Check sheet for the modelled part. Datum: model origin and axes. Units: mm. A direction names the side the tool comes from. Coordinates: 2 decimals unless noted, no trailing zeros. Order: outer loops, then holes, each group sorted by start corner. A loop starts at its lowest first (then second) coordinate and runs counter-clockwise, first axis right, second up.
from build123d import *

# Parameters (mm, degrees)
SKETCH1_W             = 140
SKETCH1_H             = 14
SKETCH1_W_2           = 180
SKETCH1_H_2           = 90
BOSS_EXTRUDE1_DEPTH   = 3
BOSS_EXTRUDE2_DEPTH   = 40
BOSS_EXTRUDE2_DRAFT   = -25
SHELL1_T              = -2
BOSS_EXTRUDE4_DEPTH   = 1.5
SCALE1_SCALE          = 0.4777778
CUT_EXTRUDE3_START    = -10
CUT_EXTRUDE3_DEPTH    = 4
SNAP_START            = -31.975695848
SNAP_HOOK1_DEPTH      = 0.247222222
SNAP_START_2          = -6.313244992
SNAP_HOOK1_2_DEPTH    = 7.314130886
SNAP_START_3          = -5.262379505
SNAP_HOOK1_3_DEPTH    = 5.212399912
SNAP_START_4          = -34
SNAP_HOOK1_4_DEPTH    = 4
SKETCH16_W            = 5
SKETCH16_H            = 1
SKETCH16_W_2          = 0.5
SKETCH16_H_2          = 3.5
SKETCH16_W_3          = 10.020724484
SKETCH16_W_4          = 6.639207239
BOSS_EXTRUDE5_DEPTH   = 10
CUT_EXTRUDE8_DEPTH    = 3.5
BOSS_EXTRUDE9_DEPTH   = 1.5
MIRROR34_START        = -31.975695848
MIRROR34_COPY_1_DEPTH = 0.247222222
MIRROR34_START_2      = -6.313244992
MIRROR34_COPY_2_DEPTH = 7.314130886
MIRROR34_START_3      = -5.262379505
MIRROR34_COPY_3_DEPTH = 5.212399912
MIRROR34_START_4      = -34
MIRROR34_COPY_4_DEPTH = 4
MIRROR34_COPY_5_DEPTH = 7.314130886
MIRROR34_COPY_6_DEPTH = 5.212399912
MIRROR34_COPY_7_DEPTH = 4
SKETCH32_R            = 1.25
CUT_EXTRUDE9_DEPTH    = 3


with BuildPart() as part:
    # Sketch1 → Boss-Extrude1 (new body)
    with BuildSketch(Plane(origin=(0, 0, 0), x_dir=(1, 0, 0), z_dir=(0, 1, 0))):
        with Locations((0, -52)):
            Rectangle(SKETCH1_W, SKETCH1_H)
        Rectangle(SKETCH1_W_2, SKETCH1_H_2)
        with Locations((0, 52)):
            Rectangle(SKETCH1_W, SKETCH1_H)
    extrude(amount=BOSS_EXTRUDE1_DEPTH)


with BuildPart() as boss_extrude2_tool:
    # Sketch2 → Boss-Extrude2 (with draft: the straight prism first)
    with BuildSketch(Plane(origin=(0, 3, 0), x_dir=(1, 0, 0), z_dir=(0, 1, 0))):
        Polygon((87, -42), (87, 42), (66, 42), (66, 56), (-66, 56), (-66, 42), (-87, 42), (-87, -42), (-65, -42), (-65, -56), (66, -56), (66, -42), align=None)
    extrude(amount=-BOSS_EXTRUDE2_DEPTH)
    # Boss-Extrude2: the draft: its side faces are tilted about the plane it starts from
    boss_extrude2_sides = [boss_extrude2_tool.faces().sort_by_distance(p)[0] for p in [
        (87, -17, 0),
        (76.5, -17, -42),
        (66, -17, -49),
        (0, -17, -56),
        (-66, -17, -49),
        (-76.5, -17, -42),
        (-87, -17, 0),
        (-76, -17, 42),
        (-65, -17, 49),
        (0.5, -17, 56),
        (66, -17, 49),
        (76.5, -17, 42),
    ]]
    draft(boss_extrude2_sides, Plane(origin=(0, 3, 0), x_dir=(1, 0, 0), z_dir=(0, 1, 0)), BOSS_EXTRUDE2_DRAFT)


with BuildPart() as part_1:
    add(part.part)

    # Boss-Extrude2: add boss_extrude2_tool
    add(boss_extrude2_tool.part)

    # Shell1
    shell1_openings = [part_1.faces().sort_by_distance(p)[0] for p in [
        (0, 3, 0),
    ]]
    offset(amount=SHELL1_T, openings=shell1_openings, kind=Kind.INTERSECTION)

    # Sketch6 → Boss-Extrude4 (add)
    with BuildSketch(Plane(origin=(0, 3, 0), x_dir=(1, 0, 0), z_dir=(0, 1, 0))):
        Polygon((94, 49), (75.612106054, 49), (75.612106054, 67), (-74.387893946, 67), (-74.387893946, 49), (-94, 49), (-94, -49), (-76, -49), (-76, -67), (74, -67), (74, -49), (94, -49), align=None)
        Polygon((88, -43), (88, 43), (68, 43), (68, 57), (-68.106730885, 57.932601668), (-68.106730885, 43), (-88, 43), (-88, -43), (-68.106730885, -43), (-68, -57), (68, -57), (68, -43), align=None, mode=Mode.SUBTRACT)
    extrude(amount=BOSS_EXTRUDE4_DEPTH)


with BuildPart() as part_2:
    # Scale1: scaled about (0.020709859, -17.532954153, 0.067819315)
    add(part_1.part.scale(SCALE1_SCALE).moved(Location((0.010815148, -9.15609789, 0.035416752))))

    # Cut-Extrude3: read off the stored shape, not the designer's step
    # Cut-Extrude3 outline → Cut-Extrude3 (cut)
    with BuildSketch(Plane(origin=(0, 0, 0), x_dir=(1, 0, 0), z_dir=(0, 1, 0)).offset(CUT_EXTRUDE3_START)):
        with BuildLine():
            ThreePointArc((-34.301389296, -32.046529352), (-35.32011541, -30.872581639), (-36.300297652, -29.666265387))
            Line((-36.300297652, -29.666265387), (-36.300297652, -32.046529352))
            Line((-36.300297652, -32.046529352), (-34.301389296, -32.046529352))
        make_face()
        with BuildLine():
            Line((-40.483605991, 23.375695448), (-44.900298052, 23.375695448))
            Line((-44.900298052, 23.375695448), (-44.900298052, 12.517856629))
            ThreePointArc((-44.900298052, 12.517856629), (-43.024636929, 18.082103779), (-40.483605991, 23.375695448))
        make_face()
        with BuildLine():
            Line((-35.530069168, 31.975695848), (-35.530069168, 30.612812124))
            ThreePointArc((-35.530069168, 30.612812124), (-34.950219267, 31.299743697), (-34.35760676, 31.975695848))
            Line((-34.35760676, 31.975695848), (-35.530069168, 31.975695848))
        make_face()
        with BuildLine():
            Line((-44.900298052, -12.525876421), (-44.900298052, -23.446528952))
            Line((-44.900298052, -23.446528952), (-40.448512682, -23.446528952))
            ThreePointArc((-40.448512682, -23.446528952), (-43.011068882, -18.123442994), (-44.900298052, -12.525876421))
        make_face()
        with BuildLine():
            Line((44.921928348, -23.446528952), (44.921928348, -20.329243571))
            ThreePointArc((44.921928348, -20.329243571), (44.151290065, -21.90247063), (43.3237572, -23.446528952))
            Line((43.3237572, -23.446528952), (44.921928348, -23.446528952))
        make_face()
        with BuildLine():
            ThreePointArc((43.35885051, 23.375695448), (44.167690984, 21.862430755), (44.921928348, 20.321223779))
            Line((44.921928348, 20.321223779), (44.921928348, 23.375695448))
            Line((44.921928348, 23.375695448), (43.35885051, 23.375695448))
        make_face()
    extrude(amount=CUT_EXTRUDE3_DEPTH, mode=Mode.SUBTRACT)



with BuildPart() as body_2:
    # Snap Hook1: read off the stored shape, not the designer's step
    # Snap Hook1 outline → Snap Hook1 (new body)
    with BuildSketch(Plane.XY.offset(SNAP_START)):
        Polygon((-5.262379505, -9.9763528), (-4.656179549, -11.2763528), (-0.656179549, -11.2763528), (-0.049979593, -9.9763528), align=None)
    snap_hook1 = extrude(amount=SNAP_HOOK1_DEPTH)


with BuildPart() as part_3:
    add(part_2.part)

    add(body_2.part)  # Snap Hook1 2 merges body 2
    # Snap Hook1 2 outline → Snap Hook1 2 (add)
    with BuildSketch(Plane.YZ.offset(SNAP_START_2)):
        Polygon((-9.9763528, -31.975695848), (-7.72276449, -31.975695848), (-7.72276449, -31.037498121), (-11.2763528, -31.728473626), (-9.9763528, -31.728473626), align=None)
    snap_hook1_2 = extrude(amount=SNAP_HOOK1_2_DEPTH)

    # Snap Hook1 3 outline → Snap Hook1 3 (add)
    with BuildSketch(Plane.YZ.offset(SNAP_START_3)):
        Polygon((-9.9763528, -32.725695848), (-9.9763528, -31.975695848), (-11.2763528, -31.975695848), (-10.2263528, -32.725695848), align=None)
    snap_hook1_3 = extrude(amount=SNAP_HOOK1_3_DEPTH)

    # Snap Hook1 4 outline → Snap Hook1 4 (cut)
    with BuildSketch(Plane.XY.offset(SNAP_START_4)):
        Polygon((-6.313244992, -7.72276449), (-6.313244992, -13), (-3.85242966, -13), (-4.656179549, -11.2763528), align=None)
        Polygon((-0.656179549, -11.2763528), (-1.459929438, -13), (1.000885894, -13), (1.000885894, -7.72276449), align=None)
    snap_hook1_4 = extrude(amount=SNAP_HOOK1_4_DEPTH, mode=Mode.SUBTRACT)

    # Sketch16 → Boss-Extrude5 (add)
    with BuildSketch(Plane(origin=(0, -25.87832089, 0), x_dir=(1, 0, 0), z_dir=(0, 1, 0))):
        with Locations((-16.965194138, 12.3890301)):
            Rectangle(SKETCH16_W, SKETCH16_H)
        with Locations((-19.715194138, 13.6390301)):
            Rectangle(SKETCH16_W_2, SKETCH16_H_2)
        with Locations((-14.454831896, 14.8890301)):
            Rectangle(SKETCH16_W_3, SKETCH16_H)
        with Locations((-0.965194138, 12.3890301)):
            Rectangle(SKETCH16_W, SKETCH16_H)
        with Locations((-1.784797758, 14.8890301)):
            Rectangle(SKETCH16_W_4, SKETCH16_H)
        Polygon((2.034805862, 15.3890301), (1.534805862, 15.3890301), (1.534805862, 14.3890301), (1.534805862, 12.8890301), (1.534805862, 11.8890301), (2.034805862, 11.8890301), align=None)
    extrude(amount=BOSS_EXTRUDE5_DEPTH)

    # Mirror17: Snap Hook1, Snap Hook1 2, Snap Hook1 3, Snap Hook1 4 across plane
    add(snap_hook1.mirror(Plane.XY))
    add(snap_hook1_2.mirror(Plane.XY))
    add(snap_hook1_3.mirror(Plane.XY))
    add(snap_hook1_4.mirror(Plane.XY), mode=Mode.SUBTRACT)

    # Sketch28 → Cut-Extrude8 (cut, symmetric)
    with BuildSketch(Plane(origin=(0, -11.613740983, -24.905747912), x_dir=(-1, 0, 0), z_dir=(0, -0.42261826174070033, -0.9063077870366497))):
        Polygon((23.440057223, -0.056353665), (15.221105561, -11.884805387), (-10.068654735, -11.884805387), (-10.068654735, -0.056353665), align=None)
    cut_extrude8 = extrude(amount=CUT_EXTRUDE8_DEPTH, both=True, mode=Mode.SUBTRACT)

    # Mirror33: Cut-Extrude8 across plane
    add(cut_extrude8.mirror(Plane.XY), mode=Mode.SUBTRACT)

    # Sketch31 → Boss-Extrude9 (add)
    with BuildSketch(Plane(origin=(12, 0, 0), x_dir=(0, 0, -1), z_dir=(1, 0, 0))):
        Polygon((-25.513843155, -8.20054229), (-17.270559615, -25.87832089), (17.199726111, -25.87832089), (25.443009652, -8.20054229), (25.443009652, -7.091787122), (-25.513843155, -7.091787122), align=None)
    extrude(amount=BOSS_EXTRUDE9_DEPTH)

    # Mirror34: Snap Hook1, Snap Hook1 2, Snap Hook1 3, Snap Hook1 4 across plane
    add(snap_hook1.mirror(Plane(origin=(12, 0, 0), x_dir=(0, 0, 1), z_dir=(1, 0, 0))))
    add(snap_hook1_2.mirror(Plane(origin=(12, 0, 0), x_dir=(0, 0, 1), z_dir=(1, 0, 0))))
    add(snap_hook1_3.mirror(Plane(origin=(12, 0, 0), x_dir=(0, 0, 1), z_dir=(1, 0, 0))))
    add(snap_hook1_4.mirror(Plane(origin=(12, 0, 0), x_dir=(0, 0, 1), z_dir=(1, 0, 0))), mode=Mode.SUBTRACT)



with BuildPart() as body_2_2:
    # Mirror34 copy 1 sketch → Mirror34 copy 1 (new body)
    with BuildSketch(Plane(origin=(24, 0, 0), x_dir=(-1, 0, 0), z_dir=(0, 0, -1)).offset(MIRROR34_START)):
        Polygon((-5.262379505, -9.9763528), (-4.656179549, -11.2763528), (-0.656179549, -11.2763528), (-0.049979593, -9.9763528), align=None)
    extrude(amount=MIRROR34_COPY_1_DEPTH)


with BuildPart() as part_4:
    add(part_3.part)

    add(body_2_2.part)  # Mirror34 copy 2 merges body 2 2
    # Mirror34 copy 2 sketch → Mirror34 copy 2 (add)
    with BuildSketch(Plane(origin=(24, 0, 0), x_dir=(0, 1, 0), z_dir=(-1, 0, 0)).offset(MIRROR34_START_2)):
        Polygon((-9.9763528, -31.975695848), (-7.72276449, -31.975695848), (-7.72276449, -31.037498121), (-11.2763528, -31.728473626), (-9.9763528, -31.728473626), align=None)
    extrude(amount=MIRROR34_COPY_2_DEPTH)

    # Mirror34 copy 3 sketch → Mirror34 copy 3 (add)
    with BuildSketch(Plane(origin=(24, 0, 0), x_dir=(0, 1, 0), z_dir=(-1, 0, 0)).offset(MIRROR34_START_3)):
        Polygon((-9.9763528, -32.725695848), (-9.9763528, -31.975695848), (-11.2763528, -31.975695848), (-10.2263528, -32.725695848), align=None)
    extrude(amount=MIRROR34_COPY_3_DEPTH)

    # Mirror34 copy 4 sketch → Mirror34 copy 4 (cut)
    with BuildSketch(Plane(origin=(24, 0, 0), x_dir=(-1, 0, 0), z_dir=(0, 0, -1)).offset(MIRROR34_START_4)):
        Polygon((-6.313244992, -7.72276449), (-6.313244992, -13), (-3.85242966, -13), (-4.656179549, -11.2763528), align=None)
        Polygon((-0.656179549, -11.2763528), (-1.459929438, -13), (1.000885894, -13), (1.000885894, -7.72276449), align=None)
    extrude(amount=MIRROR34_COPY_4_DEPTH, mode=Mode.SUBTRACT)

    # Mirror34 copy 5 sketch → Mirror34 copy 5 (add)
    with BuildSketch(Plane(origin=(24, 0, 0), x_dir=(0, 1, 0), z_dir=(-1, 0, 0)).offset(MIRROR34_START_2)):
        Polygon((-9.9763528, 31.975695848), (-7.72276449, 31.975695848), (-7.72276449, 31.037498121), (-11.2763528, 31.728473626), (-9.9763528, 31.728473626), align=None)
    extrude(amount=MIRROR34_COPY_5_DEPTH)

    # Mirror34 copy 6 sketch → Mirror34 copy 6 (add)
    with BuildSketch(Plane(origin=(24, 0, 0), x_dir=(0, 1, 0), z_dir=(-1, 0, 0)).offset(MIRROR34_START_3)):
        Polygon((-9.9763528, 32.725695848), (-9.9763528, 31.975695848), (-11.2763528, 31.975695848), (-10.2263528, 32.725695848), align=None)
    extrude(amount=MIRROR34_COPY_6_DEPTH)

    # Mirror34 copy 7 sketch → Mirror34 copy 7 (cut)
    with BuildSketch(Plane(origin=(24, 0, 0), x_dir=(-1, 0, 0), z_dir=(0, 0, 1)).offset(MIRROR34_START_4)):
        Polygon((-6.313244992, 7.72276449), (-6.313244992, 13), (-3.85242966, 13), (-4.656179549, 11.2763528), align=None)
        Polygon((-0.656179549, 11.2763528), (-1.459929438, 13), (1.000885894, 13), (1.000885894, 7.72276449), align=None)
    extrude(amount=MIRROR34_COPY_7_DEPTH, mode=Mode.SUBTRACT)

    # Sketch32 → Cut-Extrude9 (cut)
    with BuildSketch(Plane(origin=(13.5, 0, 0), x_dir=(0, 0, -1), z_dir=(1, 0, 0))):
        with Locations((0, -18.57832089)):
            Circle(SKETCH32_R)
    extrude(amount=-CUT_EXTRUDE9_DEPTH, mode=Mode.SUBTRACT)


solid = part_4.part
(1) Cross-section at D-D (x = 18). Enter the section's corners in (y, z).
Filled in:
outline: (-26.83, -17.81) - (-9.16, -26.05) - (-9.16, -28.15) - (-7.72, -28.15) - (-7.72, -31.98) - (-7.01, -31.98) - (-7.01, -27.3) - (-7.72, -27.3) - (-7.72, -27.2) - (-8.2, -27.2) - (-8.2, -25.44) - (-25.88, -17.2) - (-25.88, 17.27) - (-8.2, 25.51) - (-8.2, 27.27) - (-7.01, 27.27) - (-7.01, 32.05) - (-7.72, 32.05) - (-7.72, 28.22) - (-9.16, 28.22) - (-9.16, 26.12) - (-26.83, 17.88) - close
(2) Release check for a two-part mould opening along X. For faces 1 (the flat face through (31.64, -17.87, 15.37)), 2 (the cylindrical face through (12.76, -19.8, 0.27)), 3 (the flat face through (-36.824, -17.871, -0.236)) record: +X half, -X half, draft (parallel to the pull), parting line (faces both ways), or undercut.
Filled in:
face 1: draft
face 2: undercut
face 3: -X half
(3) Cross-section at B-B (x = 6). Count the separate pieces of the cut face and the enclosed holes in it, and give its area (3 significant figures).
Filled in:
separate pieces: 3
enclosed holes: 0
area: 60.4 mm2
(4) Go/stop test with flat-tipped pins: P1, Ø6, axis at x = 18.5, y = -13, coming from the +Z side; P2, Ø1.5, axis at x = -2, y = -20, coming from the -Z side; P3, Ø6, axis at x = -14.5, y = -24.5, coming from the -Z side. Record where each tip stops, or that it passes through.
Filled in:
P1: stops at z = 25.73
P2: stops at z = -15.39
P3: stops at z = -20.18
(5) Cross-section at A-A (z = 0). Enter the section's corners in (x, y), and give its area (3 significant figures).
Filled in:
outline: (-44.9, -7.72) - (-42.99, -7.72) - (-42.99, -9.16) - (-40.89, -9.16) - (-32.64, -26.83) - (32.67, -26.83) - (40.91, -9.16) - (43.01, -9.16) - (43.01, -7.72) - (44.92, -7.72) - (44.92, -7.01) - (42.06, -7.01) - (42.06, -8.2) - (40.3, -8.2) - (32.06, -25.88) - (13.5, -25.88) - (13.5, -19.83) - (12, -19.83) - (12, -25.88) - (-32.04, -25.88) - (-40.28, -8.2) - (-42.03, -8.2) - (-42.03, -7.01) - (-44.9, -7.01) - close; (12, -17.33) - (13.5, -17.33) - (13.5, -7.09) - (12, -7.09) - close
area: 133 mm2
(6) Thickness scan on probe 1 along Z at (x, y) = (-3, -20.5); probe 2 along X at (y, z) = (-23, -15); probe 3 along X at (y, z) = (-25, -0.5) (3 decimals). Record the ranges inside material, lowest first.
Filled in:
probe 1: z = -15.39 to -14.39, -12.89 to -11.89
probe 2: x = -24.4 to -23.34, -19.97 to -9.44, -5.1 to 2.03, 12 to 13.5, 23.37 to 24.42
probe 3: x = -33.499 to -32.445, 12 to 13.5, 32.467 to 33.521
(7) Tool access check on faces 4 (the flat face through (-31.62, -17.87, -15.3)), 5 (the flat face through (-2.71, -9.08, 31.3)), 6 (the flat face through (26.2, -16.92, 18.15)), 7 (the flat face through (-43, -7.006, 0)). Record the directions out of +Z, -Z, +X, -X, +Y, -Y that give a thin tool (end or side, any length) a straight path to the whole face; none if there is none.
Filled in:
face 4: -Z, -X, -Y
face 5: +X, -X, -Y
face 6: +Y
face 7: +Z, -Z, +X, -X, +Y
